```python
from build123d import *

# Parameters (mm, degrees)
SKETCH_1_W      = 103
SKETCH_1_H      = 81
SKETCH_1_R      = 1.65
EXTRUDE_1_DEPTH = 2.5
FILLET_1_R      = 2
EXTRUDE_START   = -30
EXTRUDE_2_DEPTH = 30
SKETCH_5_R      = 2.95
SKETCH_5_R_2    = 1.65
EXTRUDE_3_DEPTH = 4


with BuildPart() as part:
    # 草图1 → 凸台-拉伸1 (new body)
    with BuildSketch(Plane(origin=(0, 0, 0), x_dir=(1, 0, 0), z_dir=(0, 1, 0))):
        with Locations((1.5, 4.5)):
            Rectangle(SKETCH_1_W, SKETCH_1_H)
        with Locations(Location((41, 31, 0), (0, 0, 270))):
            Circle(SKETCH_1_R, mode=Mode.SUBTRACT)
        with Locations(Location((41, -31, 0), (0, 0, 270))):
            Circle(SKETCH_1_R, mode=Mode.SUBTRACT)
        with Locations(Location((-41, -31, 0), (0, 0, 270))):
            Circle(SKETCH_1_R, mode=Mode.SUBTRACT)
        with Locations(Location((-41, 31, 0), (0, 0, 270))):
            Circle(SKETCH_1_R, mode=Mode.SUBTRACT)
    extrude(amount=EXTRUDE_1_DEPTH)

    # 圆角1
    fillet_1_edges = [part.edges().sort_by_distance(p)[0] for p in [
        (-50, 1.25, -45),
        (53, 1.25, -45),
        (53, 1.25, 36),
        (-50, 1.25, 36),
    ]]
    fillet(fillet_1_edges, radius=FILLET_1_R)

    # 草图4 → 凸台-拉伸2 (add)
    with BuildSketch(Plane.XZ.offset(EXTRUDE_START)):
        with BuildLine():
            Line((51, 38.5), (-48, 38.5))
            ThreePointArc((-48, 38.5), (-51.181980515, 37.181980515), (-52.5, 34))
            Line((-52.5, 34), (-52.5, -43))
            ThreePointArc((-52.5, -43), (-51.181980515, -46.181980515), (-48, -47.5))
            Line((-48, -47.5), (51, -47.5))
            ThreePointArc((51, -47.5), (54.181980515, -46.181980515), (55.5, -43))
            Line((55.5, -43), (55.5, 34))
            ThreePointArc((55.5, 34), (54.181980515, 37.181980515), (51, 38.5))
        make_face()
        with BuildLine():
            Line((51, 36), (-48, 36))
            ThreePointArc((-48, 36), (-49.414213562, 35.414213562), (-50, 34))
            Line((-50, 34), (-50, -43))
            ThreePointArc((-50, -43), (-49.414213562, -44.414213562), (-48, -45))
            Line((-48, -45), (51, -45))
            ThreePointArc((51, -45), (52.414213562, -44.414213562), (53, -43))
            Line((53, -43), (53, 34))
            ThreePointArc((53, 34), (52.414213562, 35.414213562), (51, 36))
        make_face(mode=Mode.SUBTRACT)
    extrude(amount=EXTRUDE_2_DEPTH)

    # 草图5 → 凸台-拉伸3 (add)
    # profile 1 of 4: a face of its own
    with BuildSketch(Plane(origin=(0, 2.5, 0), x_dir=(1, 0, 0), z_dir=(0, 1, 0))):
        with Locations(Location((-41, -31, 0), (0, 0, 270))):
            Circle(SKETCH_5_R)
        with Locations(Location((-41, -31, 0), (0, 0, 270))):
            Circle(SKETCH_5_R_2, mode=Mode.SUBTRACT)
    # profile 2 of 4: a face of its own
    with BuildSketch(Plane(origin=(0, 2.5, 0), x_dir=(1, 0, 0), z_dir=(0, 1, 0))):
        with Locations(Location((41, -31, 0), (0, 0, 270))):
            Circle(SKETCH_5_R)
        with Locations(Location((41, -31, 0), (0, 0, 270))):
            Circle(SKETCH_5_R_2, mode=Mode.SUBTRACT)
    # profile 3 of 4: a face of its own
    with BuildSketch(Plane(origin=(0, 2.5, 0), x_dir=(1, 0, 0), z_dir=(0, 1, 0))):
        with Locations(Location((41, 31, 0), (0, 0, 270))):
            Circle(SKETCH_5_R)
        with Locations(Location((41, 31, 0), (0, 0, 270))):
            Circle(SKETCH_5_R_2, mode=Mode.SUBTRACT)
    # profile 4 of 4: a face of its own
    with BuildSketch(Plane(origin=(0, 2.5, 0), x_dir=(1, 0, 0), z_dir=(0, 1, 0))):
        with Locations(Location((-41, 31, 0), (0, 0, 270))):
            Circle(SKETCH_5_R)
        with Locations(Location((-41, 31, 0), (0, 0, 270))):
            Circle(SKETCH_5_R_2, mode=Mode.SUBTRACT)
    extrude(amount=EXTRUDE_3_DEPTH)


solid = part.part
```
Work out the finished part from the listing and answer in its coordinate system (mm). A direction names the side the tool comes from. Coordinates: 2 decimals unless noted, no trailing zeros. Write each loop counter-clockwise with the first axis right and the second up, starting at its lowest first coordinate (ties: lowest second). Pieces come first, ordered by that corner, then holes.
Q1. A cutting plane is placed at A-A, the plane z = -31. Give the vertices of the cut face in (x, y).
Q2. Which of the six approach directions +Z, -Z, +X, -X, +Y, -Y give full straight-line access (tool end or side, diameter ignored) to faces 1 (the face through (39.87, 4.472, 33.725)), 2 (the face through (-39.885, 3.204, -32.216))?
Q3. A cutting plane is placed at D-D, the plane x = -20.5. Give the vertices of the cut face in (y, z), then the cut area to 4 significant figures.
Q4. A cutting plane is placed at B-B, the plane y = 21.25. Give the vertices of the cut face in (x, z), then the cut area to 3 significant figures.
Q5. Find the intervals of material crossed by line 1 (X direction, y = 3, z = -31); line 2 (Z direction, x = -23.5, y = 22); line 3 (X direction, y = 2, z = 31), in increasing order.
Q6. A cutting plane is placed at C-C, the plane x = -41. Give the vertices of the cut face in (y, z), then the cut area to 3 significant figures.
Q7. Determine the mould class of faces 3 (the face through (54.217, 15.21, 37.147)), 4 (the face through (-51.217, 15.21, -46.147)), 5 (the face through (39.87, 4.472, -28.275)) for opening direction Z: released by +Z, released by -Z, zero draft, split by the parting line, or undercut.
Q8. Each of these flat-tipped pins is pushed along its axis until it touches: pin 1 Ø4 at (x, z) = (-41, -31) entering from -Y; pin 2 Ø3 at (x, z) = (-40.5, 31.5) entering from +Y; pin 3 Ø8 at (x, z) = (7, -10.5) entering from +Y. Where does it stop, or does it pass through?
Findings below:
1. outline: (-52.5, 0) - (-42.65, 0) - (-42.65, 6.5) - (-43.95, 6.5) - (-43.95, 2.5) - (-50, 2.5) - (-50, 30) - (-52.5, 30) - close; (-39.35, 0) - (39.35, 0) - (39.35, 6.5) - (38.05, 6.5) - (38.05, 2.5) - (-38.05, 2.5) - (-38.05, 6.5) - (-39.35, 6.5) - close; (42.65, 0) - (55.5, 0) - (55.5, 30) - (53, 30) - (53, 2.5) - (43.95, 2.5) - (43.95, 6.5) - (42.65, 6.5) - close
2. face 1: +Y
2. face 2: +Y, -Y
3. outline: (0, -47.5) - (30, -47.5) - (30, -45) - (2.5, -45) - (2.5, 36) - (30, 36) - (30, 38.5) - (0, 38.5) - close
3. area: 352.5 mm2
4. outline: (-52.5, -43) arc R4.5 ccw to (-48, -47.5) - (51, -47.5) arc R4.5 ccw to (55.5, -43) - (55.5, 34) arc R4.5 ccw to (51, 38.5) - (-48, 38.5) arc R4.5 ccw to (-52.5, 34) - close; hole (-50, -43) arc R2 ccw to (-48, -45) - (51, -45) arc R2 ccw to (53, -43) - (53, 34) arc R2 ccw to (51, 36) - (-48, 36) arc R2 ccw to (-50, 34) - close
4. area: 931 mm2
5. line 1: x = -52.5 to -50, -43.95 to -42.65, -39.35 to -38.05, 38.05 to 39.35, 42.65 to 43.95, 53 to 55.5
5. line 2: z = -47.5 to -45, 36 to 38.5
5. line 3: x = -52.5 to -42.65, -39.35 to 39.35, 42.65 to 55.5
6. outline: (0, -47.5) - (30, -47.5) - (30, -45) - (2.5, -45) - (2.5, -33.95) - (6.5, -33.95) - (6.5, -32.65) - (0, -32.65) - close; (0, -29.35) - (6.5, -29.35) - (6.5, -28.05) - (2.5, -28.05) - (2.5, 28.05) - (6.5, 28.05) - (6.5, 29.35) - (0, 29.35) - close; (0, 32.65) - (6.5, 32.65) - (6.5, 33.95) - (2.5, 33.95) - (2.5, 36) - (30, 36) - (30, 38.5) - (0, 38.5) - close
6. area: 357 mm2
7. face 3: released by +Z
7. face 4: released by -Z
7. face 5: undercut
8. pin 1: stops at y = 0
8. pin 2: stops at y = 6.5
8. pin 3: stops at y = 2.5
